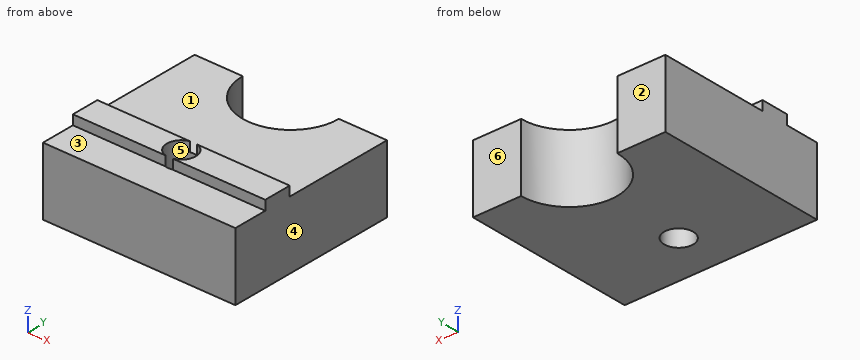
```python
from build123d import *

# Parameters (mm, degrees)
BOSS_EXTRUDE1_DEPTH = 7
SKETCH2_W           = 1
SKETCH2_H           = 2.9
BOSS_EXTRUDE2_DEPTH = 20
SKETCH3_R           = 1.5
CUT_EXTRUDE1_DEPTH  = 9


with BuildPart() as part:
    # Sketch1 → Boss-Extrude1 (new body)
    with BuildSketch(Plane.XY):
        with BuildLine():
            Line((-10, 0), (10, 0))
            Line((10, 0), (10, 18))
            Line((10, 18), (5, 18))
            ThreePointArc((5, 18), (0, 13), (-5, 18))
            Line((-5, 18), (-10, 18))
            Line((-10, 18), (-10, 0))
        make_face()
    extrude(amount=BOSS_EXTRUDE1_DEPTH)

    # Sketch2 → Boss-Extrude2 (add)
    with BuildSketch(Plane.ZY.offset(10)):
        with Locations((7.5, 5)):
            Rectangle(SKETCH2_W, SKETCH2_H)
    extrude(amount=-BOSS_EXTRUDE2_DEPTH)

    # Sketch3 → Cut-Extrude1 (cut, through all)
    with BuildSketch(Plane.XY.offset(8)):
        with Locations((0, 5)):
            Circle(SKETCH3_R)
    extrude(amount=-CUT_EXTRUDE1_DEPTH, mode=Mode.SUBTRACT)


solid = part.part
```
Could you check a few things on this model? Use its own coordinates, in mm. Face numbers are marked on the shaded views. A direction names the side the tool comes from. Round coordinates to 2 decimals unless told otherwise and drop trailing zeros. Loops run counter-clockwise (first coordinate to the right, second up) from the corner with the lowest first, then second, coordinate; pieces in that order, holes last.
Q1. I want a section at B-B (z = 1.25). Write out the boundary of the cut face in (x, y).
Q2. Thinking about a two-plate mould opening in X: for the marked faces 4, 5 and 6, which applies, pulls with the +X half, pulls with the -X half, needs draft (parallel to the pull), parting line crosses it, or undercut?
Q3. For P1, Ø1, axis at x = 8, y = 2.5, coming from the +Z side, with a flat end and sliding along its axis, tell me the tip position at first contact or that it passes through.
Q4. I want a section at A-A (y = 5). Write out the boundary of the cut face in (x, z).
Q5. Please list where these lines run through material, in increasing order: L1, parallel to Y at x = 0, z = 5.25; L2, parallel to Z at x = 6.25, y = 2; L3, parallel to X at y = 4.25, z = 5.25.
Q6. I want a section at D-D (x = -7.75). Write out the boundary of the cut face in (y, z).
Q7. On a 3-axis mill with a long thin cutter (end or side, diameter ignored), from which of +Z, -Z, +X, -X, +Y, -Y can I reach the whole of each face in a straight line? I mean the marked faces 1, 2 and 3. Say none if no direction works.
Q8. I want a section at C-C (x = 0). Write out the boundary of the cut face in (y, z).
Answer below:
1. outline: (-10, 0) - (10, 0) - (10, 18) - (5, 18) arc R5 cw to (-5, 18) - (-10, 18) - close; hole circle Ø3 at (0, 5)
2. face 4: pulls with the +X half
2. face 5: undercut
2. face 6: needs draft
3. P1: stops at z = 7
4. outline: (-10, 0) - (-1.5, 0) - (-1.5, 8) - (-10, 8) - close; (1.5, 0) - (10, 0) - (10, 8) - (1.5, 8) - close
5. L1: y = 0 to 3.5, 6.5 to 13
5. L2: z = 0 to 7
5. L3: x = -10 to -1.3, 1.3 to 10
6. outline: (0, 0) - (18, 0) - (18, 7) - (6.45, 7) - (6.45, 8) - (3.55, 8) - (3.55, 7) - (0, 7) - close
7. face 1: +Z, +X, -X, +Y
7. face 2: +Z, -Z, +X, -X, +Y
7. face 3: +Z, +X, -X, -Y
8. outline: (0, 0) - (3.5, 0) - (3.5, 7) - (0, 7) - close; (6.5, 0) - (13, 0) - (13, 7) - (6.5, 7) - close
